```python
from build123d import *

# Parameters (mm, degrees)
BOSS_EXTRUDE1_DEPTH = 170.18
SKETCH2_W           = 107.442
SKETCH2_H           = 53.34
CUT_EXTRUDE1_DEPTH  = 170.18
SKETCH3_W           = 46.821602836
SKETCH3_H           = 2.401895457
BOSS_EXTRUDE2_DEPTH = 8.1534
SKETCH4_R           = 1.4224
CUT_EXTRUDE2_DEPTH  = 10.16


with BuildPart() as part:
    # Sketch1 → Boss-Extrude1 (new body)
    with BuildSketch(Plane.XY):
        Polygon((189.487065503, 0), (177.644123909, 0), (0, 190.5), (0, 203.2), align=None)
    extrude(amount=BOSS_EXTRUDE1_DEPTH)

    # Sketch2 → Cut-Extrude1 (cut)
    with BuildSketch(Plane(origin=(101.352507506, 94.512742268, 0), x_dir=(0, 0, -1), z_dir=(0.7313537016191667, 0.6819983600625027, 0))):
        with Locations((-116.459, 59.711072169)):
            Rectangle(SKETCH2_W, SKETCH2_H)
    extrude(amount=-CUT_EXTRUDE1_DEPTH, mode=Mode.SUBTRACT)

    # Sketch3 → Boss-Extrude2 (add)
    with BuildSketch(Plane(origin=(101.352507506, 94.512742268, 0), x_dir=(0, 0, -1), z_dir=(0.7313537016191667, 0.6819983600625027, 0))):
        with Locations((-86.148801418, 34.242019898)):
            Rectangle(SKETCH3_W, SKETCH3_H)
    extrude(amount=-BOSS_EXTRUDE2_DEPTH)

    # Sketch4 → Cut-Extrude2 (cut)
    with BuildSketch(Plane.XY.offset(170.18)):
        with Locations((25.928493761, 169.045094592)):
            Circle(SKETCH4_R)
        with Locations((101.282492565, 88.2378241)):
            Circle(SKETCH4_R)
        with Locations((118.60525091, 69.661440079)):
            Circle(SKETCH4_R)
    cut_extrude2 = extrude(amount=-CUT_EXTRUDE2_DEPTH, mode=Mode.SUBTRACT)

    # Mirror1: Cut-Extrude2 across plane
    add(cut_extrude2.mirror(Plane.XY.offset(85.09)), mode=Mode.SUBTRACT)


solid = part.part
```
Geometry: final body of the model. Coordinates: model frame, mm. A direction names the side the tool comes from. Round coordinates to 2 decimals unless told otherwise and drop trailing zeros. Order: outer loops, then holes, each group sorted by start corner. A loop starts at its lowest first (then second) coordinate and runs counter-clockwise, first axis right, second up. Notation, with made-up numbers: (-4, 58.5) -> (34, 58.5) arc R23 ccw to (34, 84.5) -> close; hole circle Ø8 at (-33, 57). An arc over 180 degrees is marked (long way). Write each question's results on one line, items separated by ' | '.
Q1. Section query A-A (z = 78.5). Output: boundary loops of the cut face in (x, y).
Response values:
outline: (0, 190.5) -> (36.11, 151.78) -> (42.44, 157.69) -> (0, 203.2) -> close; (71.22, 114.87) -> (72.86, 113.12) -> (72.48, 112.77) -> (177.64, 0) -> (189.49, 0) -> (77.18, 120.43) -> close
Q2. Section query D-D (x = 113.5). Output: boundary loops of the cut face in (y, z), and give its area (3 significant figures).
Response values:
outline: (68.79, 0) -> (81.49, 0) -> (81.49, 170.18) -> (68.79, 170.18) -> close | area: 2,160 mm²
Q3. Section query B-B (z = 129.5). Output: boundary loops of the cut face in (x, y).
Response values:
outline: (0, 190.5) -> (36.11, 151.78) -> (42.44, 157.69) -> (0, 203.2) -> close; (72.48, 112.77) -> (177.64, 0) -> (189.49, 0) -> (78.82, 118.68) -> close
Q4. Pin query (flat end, axial travel): pin 1 Ø0.9 at (x, y) = (26, 169.5) entering from -Z; pin 2 Ø1.5 at (y, z) = (131, 65) entering from +X; pin 3 Ø4 at (y, z) = (92, 36.5) entering from +X; pin 4 Ø6 at (y, z) = (27.5, 18.5) entering from -X. Return the tip coordinate at first contact, or that it passes through.
Response values:
pin 1: z = 10.16 | pin 2: through | pin 3: x = 105.56 | pin 4: x = 149.2
Q5. Ray query, line 1 along X through (y, z) = (23, 51); line 2 along Y through (x, z) = (89.5, 148); line 3 along Y through (x, z) = (39.5, 54.5). Return the intervals inside material, ascending.
Response values:
line 1: 156.2 to 168.04 | line 2: 94.52 to 107.22 | line 3: 148.14 to 160.84
Q6. Section query C-C (y = 54). Output: boundary loops of the cut face in (x, z).
Response values:
outline: (127.29, 0) -> (139.13, 0) -> (139.13, 170.18) -> (127.29, 170.18) -> close
Q7. Access query for faces 1 (the face through (39.32, 154.78, 117.21)), 2 (the face through (75, 117, 109.56)), 3 (the face through (95, 95, 0)). Directions: +Z, -Z, +X, -X, +Y, -Y. A direction counts if a zero-diameter tool reaches every point of the face in a straight line with its end or side. Return the directions, or none.
Response values:
face 1: +Z, +X, -Y | face 2: +Z, -X, +Y | face 3: -Z, +X, -X, +Y, -Y
